Verification items for the finished model (mm, model axes). A direction names the side the tool comes from. Round coordinates to 2 decimals unless told otherwise and drop trailing zeros. Write each loop counter-clockwise with the first axis right and the second up, starting at its lowest first coordinate (ties: lowest second). Pieces come first, ordered by that corner, then holes. Notation, with made-up numbers: M 12,-21 L 31,-21 A30 ccw 31,10 Z; hole C 61.5,75 d6. An arc over 180 degrees is marked long. Answer in a Markdown table with one row per item. Add a question column.
1. Sectioned sample at C-C on z = -13. Record the cut outline in (x, y).
2. Draft check along X on faces 6 (the flat face through (0, -73.914, -4)), 7 (the flat face through (0, -37, 6.35)), 8 (the cylindrical face through (-13.858, -36.44, -10.626)), 9 (the flat face through (-4.762, -83, -6)). Enter one of: pulls with the +X half, pulls with the -X half, needs draft (parallel to the pull), parting line crosses it, or undercut.
3. Material ranges on probe 1 along Y at (x, z) = (-7, 8.5); probe 2 along Z at (x, y) = (2, -39.5); probe 3 along Z at (x, y) = (-4, -15.5), recorded low to high.
4. Sectioned sample at A-A on x = 0. Record the cut outline in (y, z).
5. Sectioned sample at D-D on x = -11. Record the cut outline in (y, z), plus the area to 3 significant figures.
6. Go/stop test with flat-tipped pins: pin 1 Ø1 at (y, z) = (-85.5, -7) entering from +X; pin 2 Ø3 at (x, y) = (-5, -70.5) entering from +Z; pin 3 Ø5 at (x, z) = (13.5, -3) entering from +Y; pin 4 Ø4 at (x, z) = (10, 8) entering from -Y. Record where each tip stops, or that it passes through.
7. Set-up check for faces 1 (the flat face through (0, -37, 0)), 2 (the flat face through (0, -83, -7.938)), 3 (the flat face through (4.762, -83, -6)), 4 (the flat face through (0, -92.964, -6)), 5 (the flat face through (0, -83, -4.762)): record each of +Z, -Z, +X, -X, +Y, -Y from which the full face is reachable in a straight line by a thin tool's end or side.
```python
from build123d import *

# Parameters (mm, degrees)
F0_R     = 17.4625
F1_DEPTH = 73.914
F2_W     = 12.7
F2_H     = 6.35
F3_DEPTH = 178.054
F4_W     = 9.525
F4_H     = 3.175
F5_DEPTH = 19.05


with BuildPart() as f1:
    # F0 (on Front) → F1 (new body)
    with BuildSketch(Plane.XZ):
        Circle(F0_R)
    extrude(amount=F1_DEPTH)

    # F2 (on face) → F3 (cut)
    with BuildSketch(Plane.XZ.offset(73.914)):
        with Locations((0, 3.175)):
            Rectangle(F2_W, F2_H)
    extrude(amount=-F3_DEPTH, mode=Mode.SUBTRACT)

    # F4 (on face) → F5 (join)
    with BuildSketch(Plane.XZ.offset(73.914)):
        with Locations((0, -6.35)):
            Rectangle(F4_W, F4_H)
    extrude(amount=F5_DEPTH)


solid = f1.part
```
Geometry check:
| question | item | result |
|---|---|---|
| 1 | outline | M -11.66,-73.91 L 11.66,-73.91 L 11.66,0 L -11.66,0 Z |
| 2 | face 6 | needs draft |
| 2 | face 7 | undercut |
| 2 | face 8 | parting line crosses it |
| 2 | face 9 | pulls with the -X half |
| 3 | probe 1 | y = -73.91 to 0 |
| 3 | probe 2 | z = -17.35 to 0, 6.35 to 17.35 |
| 3 | probe 3 | z = -17 to 0, 6.35 to 17 |
| 4 | outline | M -92.96,-7.94 L -73.91,-7.94 L -73.91,-17.46 L 0,-17.46 L 0,0 L -73.91,0 L -73.91,-4.76 L -92.96,-4.76 Z; M -73.91,6.35 L 0,6.35 L 0,17.46 L -73.91,17.46 Z |
| 5 | outline | M -73.91,-13.56 L 0,-13.56 L 0,13.56 L -73.91,13.56 Z |
| 5 | area | 2,000 mm2 |
| 6 | pin 1 | stops at x = 4.76 |
| 6 | pin 2 | stops at z = 17.11 |
| 6 | pin 3 | stops at y = 0 |
| 6 | pin 4 | stops at y = -73.91 |
| 7 | face 1 | +Y, -Y |
| 7 | face 2 | -Z, +X, -X, -Y |
| 7 | face 3 | +Z, -Z, +X, -Y |
| 7 | face 4 | +Z, -Z, +X, -X, -Y |
| 7 | face 5 | +Z, +X, -X, -Y |
